from build123d import *

# Parameters (mm, degrees)
F0_W     = 45
F0_H     = 35
F1_DEPTH = 7.5
F2_W     = 40
F2_H     = 30
F3_DEPTH = 7.5
F4_W     = 40
F4_H     = 30
F5_DEPTH = 5
F6_R     = 5


with BuildPart() as f1:
    # F0 (on Top) → F1 (new body, symmetric)
    with BuildSketch(Plane.XY):
        Rectangle(F0_W, F0_H)
    extrude(amount=F1_DEPTH, both=True)

    # F2 (on Top) → F3 (cut)
    with BuildSketch(Plane.XY):
        Rectangle(F2_W, F2_H)
    extrude(amount=F3_DEPTH, mode=Mode.SUBTRACT)

    # F4 (on Top) → F5 (join)
    with BuildSketch(Plane.XY):
        Rectangle(F4_W, F4_H)
    extrude(amount=-F5_DEPTH)

    # F6
    f6_edges = [f1.edges().sort_by_distance(p)[0] for p in [
        (20, 15, 3.75),
        (-20, 15, 3.75),
        (-20, -15, 3.75),
        (20, -15, 3.75),
    ]]
    fillet(f6_edges, radius=F6_R)


solid = f1.part
Can you work these out from the model? Positions are in its coordinate system, mm. A direction names the side the tool comes from. Round coordinates to 2 decimals unless told otherwise and drop trailing zeros. Order: outer loops, then holes, each group sorted by start corner. A loop starts at its lowest first (then second) coordinate and runs counter-clockwise, first axis right, second up. Notation, with made-up numbers: (-11.5, -11.5) -> (0.5, -11.5) arc R31 cw to (0.5, 23.5) -> close; hole circle Ø5 at (50.5, -31). An arc over 180 degrees is marked (long way). Write each question's results on one line, items separated by ' | '. Start each with the question number.
Item 1: If we section it at B-B, the plane z = 1: Write out the boundary of the cut face in (x, y).
Item 2: Will this pin go through, and if not, where does the flat tip stop? pin 1 (2 mm diameter, centred on x = -16, y = -8.5, fed in from +Z).
Item 3: Thinking about a two-plate mould opening in X: for faces 3 (the cylindrical face through (19, 13, 4)), 4 (the flat face through (22.5, 0, 0)), 5 (the flat face through (0, 0, -7.5)), which applies, +X half, -X half, draft (parallel to the pull), parting line (faces both ways), or undercut?
Item 4: If we section it at A-A, the plane y = -13: Write out the boundary of the cut face in (x, z).
Item 5: Please list where these lines run through material, in increasing order: L1, parallel to Y at x = 7.5, z = 4; L2, parallel to X at y = -9.5, z = 5; L3, parallel to Y at x = 17.5, z = 2.5.
Item 6: Which directions (+Z, -Z, +X, -X, +Y, -Y) give clear straight access to the entire face, cutting with the end or side of a thin tool? Please do faces 1 (the cylindrical face through (-19, -13, 4)), 2 (the flat face through (0, 17.5, 0)).
Item 7: If we section it at C-C, the plane x = -19: Write out the boundary of the cut face in (y, z), then the cut area to 3 significant figures.
Results:
1) outline: (-22.5, -17.5) -> (22.5, -17.5) -> (22.5, 17.5) -> (-22.5, 17.5) -> close; hole (-20, -10) arc R5 ccw to (-15, -15) -> (15, -15) arc R5 ccw to (20, -10) -> (20, 10) arc R5 ccw to (15, 15) -> (-15, 15) arc R5 ccw to (-20, 10) -> close
2) pin 1: stops at z = 0
3) face 3: undercut | face 4: +X half | face 5: draft
4) outline: (-22.5, -7.5) -> (22.5, -7.5) -> (22.5, 7.5) -> (19, 7.5) -> (19, 0) -> (-19, 0) -> (-19, 7.5) -> (-22.5, 7.5) -> close
5) L1: y = -17.5 to -15, 15 to 17.5 | L2: x = -22.5 to -20, 20 to 22.5 | L3: y = -17.5 to -14.33, 14.33 to 17.5
6) face 1: +Z | face 2: +Z, -Z, +X, -X, +Y
7) outline: (-17.5, -7.5) -> (17.5, -7.5) -> (17.5, 7.5) -> (13, 7.5) -> (13, 0) -> (-13, 0) -> (-13, 7.5) -> (-17.5, 7.5) -> close | area: 330 mm2
